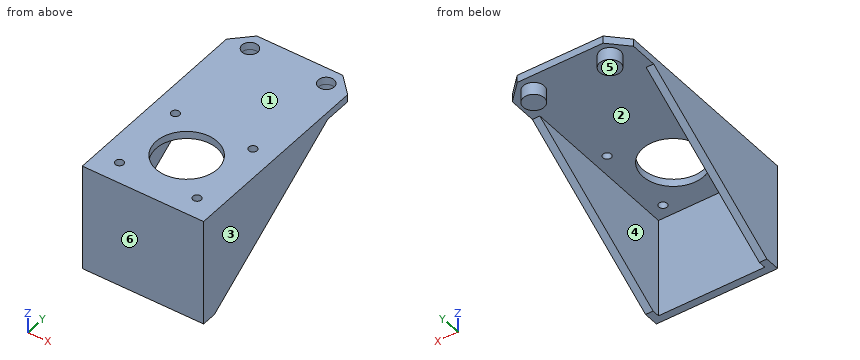
from build123d import *
from build123d.topology import SkipClean

# Parameters (mm, degrees)
SKETCH1_R                = 1.65
SKETCH1_R_2              = 12.25
SKETCH1_R_3              = 3.175
BOSS_EXTRUDE1_DEPTH      = 3
BOSS_EXTRUDE2_START      = 3
SKETCH2_R                = 4.175
SKETCH2_R_2              = 3.175
BOSS_EXTRUDE2_DEPTH      = 3
BOSS_EXTRUDE3_START      = 2
SKETCH3_R                = 4.175
BOSS_EXTRUDE3_DEPTH      = 2
BOSS_EXTRUDE4_DEPTH      = 40
BOSS_EXTRUDE4_DEPTH_BACK = 3
SKETCH5_W                = 3
SKETCH5_H                = 5
BOSS_EXTRUDE5_DEPTH      = 3
BOSS_EXTRUDE7_DEPTH      = 3
BOSS_EXTRUDE9_DEPTH      = 3
SKETCH9_W                = 3
SKETCH9_H                = 75.55
BOSS_EXTRUDE10_DEPTH     = 3
CHAMFER1_SIZE            = 3
BOSS_EXTRUDE12_DEPTH     = 3
BOSS_EXTRUDE13_DEPTH     = 3
BOSS_EXTRUDE14_DEPTH     = 3


with BuildPart() as part:
    # Sketch1 → Boss-Extrude1 (new body)
    with BuildSketch(Plane.XY):
        Polygon((-33.82227566, -6), (-33.82227566, 36.5), (-33.82227566, 72.55), (-28.82227566, 77.55), (3.67772434, 77.55), (8.67772434, 72.55), (8.67772434, 36.5), (8.67772434, -6), align=None)
        with Locations((2.92772434, 30.5)):
            Circle(SKETCH1_R, mode=Mode.SUBTRACT)
        with Locations(Location((2.92772434, -0.5, 0), (0, 0, 180))):
            Circle(SKETCH1_R, mode=Mode.SUBTRACT)
        with Locations((-28.07227566, -0.5)):
            Circle(SKETCH1_R, mode=Mode.SUBTRACT)
        with Locations(Location((-28.07227566, 30.5, 0), (0, 0, 180))):
            Circle(SKETCH1_R, mode=Mode.SUBTRACT)
        with Locations((-12.57227566, 15.25)):
            Circle(SKETCH1_R_2, mode=Mode.SUBTRACT)
        with Locations((-27.82227566, 71.55)):
            Circle(SKETCH1_R_3, mode=Mode.SUBTRACT)
        with Locations(Location((2.67772434, 71.55, 0), (0, 0, 180))):
            Circle(SKETCH1_R_3, mode=Mode.SUBTRACT)
    extrude(amount=BOSS_EXTRUDE1_DEPTH)

    # Sketch2 → Boss-Extrude2 (add)
    # profile 1 of 2: a face of its own
    with SkipClean():  # the faces are left unmerged after this step: merging them gives an invalid solid
        with BuildSketch(Plane(origin=(0, 0, 0), x_dir=(-1, 0, 0), z_dir=(0, 0, -1)).offset(BOSS_EXTRUDE2_START)):
            with Locations((-2.67772434, 71.55)):
                Circle(SKETCH2_R)
            with Locations((-2.67772434, 71.55)):
                Circle(SKETCH2_R_2, mode=Mode.SUBTRACT)
        # profile 2 of 2: a face of its own
        with BuildSketch(Plane(origin=(0, 0, 0), x_dir=(-1, 0, 0), z_dir=(0, 0, -1)).offset(BOSS_EXTRUDE2_START)):
            with Locations((27.82227566, 71.55)):
                Circle(SKETCH2_R)
            with Locations((27.82227566, 71.55)):
                Circle(SKETCH2_R_2, mode=Mode.SUBTRACT)
        extrude(amount=-BOSS_EXTRUDE2_DEPTH)

    # Sketch3 → Boss-Extrude3 (add)
    with SkipClean():  # the faces are left unmerged after this step: merging them gives an invalid solid
        with BuildSketch(Plane(origin=(0, 0, -3), x_dir=(-1, 0, 0), z_dir=(0, 0, -1)).offset(BOSS_EXTRUDE3_START)):
            with Locations((-2.67772434, 71.55)):
                Circle(SKETCH3_R)
            with Locations((27.82227566, 71.55)):
                Circle(SKETCH3_R)
        extrude(amount=-BOSS_EXTRUDE3_DEPTH)

    # Sketch5 → Boss-Extrude5 (add)
    with SkipClean():  # the faces are left unmerged after this step: merging them gives an invalid solid
        with BuildSketch(Plane.XY.offset(3)):
            with Locations((10.17772434, 45.531399611)):
                Rectangle(SKETCH5_W, SKETCH5_H)
            with Locations((-35.32227566, 45.531399611)):
                Rectangle(SKETCH5_W, SKETCH5_H)
        extrude(amount=-BOSS_EXTRUDE5_DEPTH)



with BuildPart() as body_2:
    # Sketch4 → Boss-Extrude4 (new, two sides: drawn at the far end of the back side and taken through both)
    with BuildSketch(Plane(origin=(0, 0, 0), x_dir=(-1, 0, 0), z_dir=(0, 0, -1)).offset(-BOSS_EXTRUDE4_DEPTH_BACK)):
        Polygon((33.82227566, -6), (-8.67772434, -6), (-8.67772434, -3), (-11.67772434, -3), (-11.67772434, -9), (-9.078713654, -9), (33.421286346, -9), (36.82227566, -9), (36.82227566, -3), (33.82227566, -3), align=None)
    extrude(amount=BOSS_EXTRUDE4_DEPTH + BOSS_EXTRUDE4_DEPTH_BACK)


with BuildPart() as part_1:
    with SkipClean():  # the faces are left unmerged after this step: merging them gives an invalid solid
        add(part.part)

        add(body_2.part)  # Boss-Extrude7 merges body 2
        # Sketch6 → Boss-Extrude7 (add)
        with BuildSketch(Plane(origin=(8.67772434, 0, 0), x_dir=(0, 0, -1), z_dir=(1, 0, 0))):
            Polygon((0, 48.031399611), (40, -3), (36.080844313, -3), (0, 43.031399611), align=None)
        extrude(amount=BOSS_EXTRUDE7_DEPTH)

    # Sketch8 → Boss-Extrude9 (add)
    with SkipClean():  # the faces are left unmerged after this step: merging them gives an invalid solid
        with BuildSketch(Plane.ZY.offset(36.82227566)):
            Polygon((0, 48.031399611), (0, 43.031399611), (-36.080844313, -3), (-40, -3), align=None)
        extrude(amount=-BOSS_EXTRUDE9_DEPTH)

    # Sketch9 → Boss-Extrude10 (add)
    with SkipClean():  # the faces are left unmerged after this step: merging them gives an invalid solid
        with BuildSketch(Plane.XY.offset(3)):
            with Locations((-35.32227566, 34.775)):
                Rectangle(SKETCH9_W, SKETCH9_H)
            with Locations((10.17772434, 34.775)):
                Rectangle(SKETCH9_W, SKETCH9_H)
        extrude(amount=-BOSS_EXTRUDE10_DEPTH)

    # Chamfer1
    chamfer1_edges = [part_1.edges().sort_by_distance(p)[0] for p in [
        (11.67772434, 72.55, 1.5),
        (-36.82227566, 72.55, 1.5),
    ]]
    chamfer(chamfer1_edges, length=CHAMFER1_SIZE - 0.0001)  # a hair under: the kernel refuses the full size

    # Sketch10 → Boss-Extrude12 (add)
    with BuildSketch(Plane(origin=(11.67772434, 0, 0), x_dir=(0, 0, -1), z_dir=(1, 0, 0))):
        Polygon((-3, 64.55), (-3, -9), (40, -9), (40, -3), align=None)
    extrude(amount=-BOSS_EXTRUDE12_DEPTH)

    # Sketch11 → Boss-Extrude13 (add)
    with BuildSketch(Plane.ZY.offset(36.82227566)):
        Polygon((3, -9), (3, 64.55), (-40, -3), (-40, -9), align=None)
    extrude(amount=-BOSS_EXTRUDE13_DEPTH)

    # Sketch12 → Boss-Extrude14 (add)
    with BuildSketch(Plane.XY.offset(3)):
        Polygon((-36.82227566, 70.964213562), (-36.82227566, 69.55), (-33.82227566, 72.55), (-28.82227566, 77.55), (-12.57227566, 77.55), (-12.57227566, 78.05), (-29.736489222, 78.05), align=None)
        Polygon((4.591937902, 78.05), (-12.57227566, 78.05), (-12.57227566, 77.55), (3.67772434, 77.55), (8.67772434, 72.55), (11.67772434, 69.55), (11.67772434, 70.964213562), align=None)
    extrude(amount=-BOSS_EXTRUDE14_DEPTH)


solid = part_1.part
Geometry: final body of the model. Coordinates: model frame, mm. Face numbers are marked on the shaded views. A direction names the side the tool comes from. Give positions to 0.01 mm unless a question says otherwise; leave off trailing zeros. Loops run counter-clockwise (first coordinate to the right, second up) from the corner with the lowest first, then second, coordinate; pieces in that order, holes last. Notation, with made-up numbers: (28, 28) - (87, 28) arc R8 cw to (87, 37) - close; hole circle Ø10 at (71.25, 83.25). An arc over 180 degrees is marked (long way). One line per question, with ' | ' between items. Start each with the question number.
(1) Section query D-D on z = -23.5. Return loops of the section in (x, y), then the cut area to 3 significant figures.
(2) Ray query, line 1 (X direction, y = 15.5, z = -27); line 2 (X direction, y = 71, z = -1); line 3 (X direction, y = 71.55, z = 1.3). Return the intervals inside material, ascending. Write a range as from..to.
(3) Pull-direction query (X, two-part tool) for the marked faces 1, 2 and 3; classes: released by +X, released by -X, zero draft, split by the parting line, or undercut.
(4) Reachability of the marked faces 4, 5 and 6 from +Z, -Z, +X, -X, +Y, -Y: full face, straight path, thin tool, end or side. Return the list, or none.
(5) Section query B-B on x = -4. Return loops of the section in (y, z).
(6) Contact query for flat-ended pins moving along their axis: pin 1 (4 mm diameter, centred on x = 4.5, y = 70, fed in from -Z); pin 2 (3 mm diameter, centred on x = -26.5, y = 72, fed in from +Z); pin 3 (12 mm diameter, centred on x = -25, z = -26, fed in from +Y); pin 4 (2.5 mm diameter, centred on x = -28.07, y = -0.5, fed in from +Z). Output: stop coordinate, or through.
(7) Section query C-C on y = 30.5. Return loops of the section in (x, z).
(8) Section query A-A on y = 15.25. Return loops of the section in (x, z).
The answers:
1) outline: (-36.82, -9) - (11.68, -9) - (11.68, 22.92) - (8.68, 22.92) - (8.68, -6) - (-33.82, -6) - (-33.82, 22.92) - (-36.82, 22.92) - close | area: 319 mm2
2) line 1: -36.82..-33.82, 8.68..11.68 | line 2: -31.96..-30.95, -24.7..-23.68, -1.46..-0.45, 5.8..6.82 | line 3: -36.24..-31, -24.65..-0.5, 5.85..11.09
3) face 1: zero draft | face 2: undercut | face 3: released by +X
4) face 4: -Z, +Y | face 5: -Z, +X, -X, +Y | face 6: +Z, -Z, +X, -X, -Y
5) outline: (-9, -40) - (-6, -40) - (-6, 0) - (6.5, 0) - (6.5, 3) - (-9, 3) - close; (24, 0) - (78.05, 0) - (78.05, 3) - (24, 3) - close
6) pin 1: z = -5 | pin 2: z = -3 | pin 3: y = -6 | pin 4: through
7) outline: (-36.82, -18.68) - (-33.82, -18.68) - (-33.82, 0) - (-29.72, 0) - (-29.72, 3) - (-36.82, 3) - close; (-26.42, 0) - (1.28, 0) - (1.28, 3) - (-26.42, 3) - close; (4.58, 0) - (8.68, 0) - (8.68, -18.68) - (11.68, -18.68) - (11.68, 3) - (4.58, 3) - close
8) outline: (-36.82, -28.38) - (-33.82, -28.38) - (-33.82, 0) - (-24.82, 0) - (-24.82, 3) - (-36.82, 3) - close; (-0.32, 0) - (8.68, 0) - (8.68, -28.38) - (11.68, -28.38) - (11.68, 3) - (-0.32, 3) - close
